```python
from build123d import *

# Parameters (mm, degrees)
BOSS_EXTRUDE1_DEPTH = 12.7
SKETCH2_R           = 3.175
BOSS_EXTRUDE2_DEPTH = 84.328


with BuildPart() as part:
    # Sketch1 → Boss-Extrude1 (new body)
    with BuildSketch(Plane.XY):
        with BuildLine():
            Line((-38.1, 0), (-38.1, 51.682449807))
            Line((-38.1, 51.682449807), (38.1, 51.682449807))
            Line((38.1, 51.682449807), (38.1, 0))
            ThreePointArc((38.1, 0), (0, -38.1), (-38.1, 0))
        make_face()
    extrude(amount=BOSS_EXTRUDE1_DEPTH)

    # Sketch2 → Boss-Extrude2 (add)
    with BuildSketch(Plane(origin=(0, 0, 0), x_dir=(1, 0, 0), z_dir=(0, 1, 0))):
        with Locations(Location((0, -7.032046272, 0), (0, 0, 90))):
            Circle(SKETCH2_R)
    extrude(amount=BOSS_EXTRUDE2_DEPTH)


solid = part.part
```
Source: CAD feature listing. Evaluate the final solid. Frame: model axes, mm. A direction names the side the tool comes from. Round coordinates to 2 decimals unless told otherwise and drop trailing zeros. Loops run counter-clockwise (first coordinate to the right, second up) from the corner with the lowest first, then second, coordinate; pieces in that order, holes last.
1. Section query B-B on z = 8.5. Output: boundary loops of the cut face in (x, y).
2. Contact query for flat-ended pins moving along their axis: pin 1 (3 mm diameter, centred on x = 17, z = 8.5, fed in from -Y); pin 2 (5 mm diameter, centred on x = 22.5, z = 5, fed in from -Y). Output: stop coordinate, or through.
3. Section query A-A on x = 0. Output: boundary loops of the cut face in (y, z), and give its area (3 significant figures).
4. Ray query, L1, parallel to Y at x = 1, z = 4.5; L2, parallel to Y at x = -25, z = 7.5; L3, parallel to X at y = -3.5, z = 5. Return the intervals inside material, ascending.
5. Access query for faces 1 (the cylindrical face through (0.84, -38.09, 6.26)), 2 (the cylindrical face through (1.932, 67.777, 9.552)). Directions: +Z, -Z, +X, -X, +Y, -Y. A direction counts if a zero-diameter tool reaches every point of the face in a straight line with its end or side. Return the directions, or none.
6. Section query C-C on y = 69.5. Output: boundary loops of the cut face in (x, z) (3 decimals), and give its area (3 significant figures).
7. Section query D-D on z = 1.75. Output: boundary loops of the cut face in (x, y).
Answers below:
1. outline: (-38.1, 0) arc R38.1 ccw to (38.1, 0) - (38.1, 51.68) - (2.82, 51.68) - (2.82, 84.33) - (-2.82, 84.33) - (-2.82, 51.68) - (-38.1, 51.68) - close
2. pin 1: stops at y = -34.8
2. pin 2: stops at y = -32.43
3. outline: (-38.1, 0) - (51.68, 0) - (51.68, 3.86) - (84.33, 3.86) - (84.33, 10.21) - (51.68, 10.21) - (51.68, 12.7) - (-38.1, 12.7) - close
3. area: 1,350 mm2
4. L1: y = -38.09 to 84.33
4. L2: y = -28.75 to 51.68
4. L3: x = -37.94 to 37.94
5. face 1: +Z, -Z, -Y
5. face 2: +Y
6. outline: circle Ø6.35 at (0, 7.032)
6. area: 31.7 mm2
7. outline: (-38.1, 0) arc R38.1 ccw to (38.1, 0) - (38.1, 51.68) - (-38.1, 51.68) - close
